from build123d import *

# Parameters (mm, degrees)
SKETCH_1_W          = 30
SKETCH_1_H          = 30
SKETCH_1_W_2        = 28
SKETCH_1_H_2        = 28
EXTRUDE_1_DEPTH     = 225
SKETCH_2_R          = 2
CUT_EXTRUDE_1_DEPTH = 65
SKETCH_4_R          = 2
CUT_EXTRUDE_2_DEPTH = 45
SKETCH_5_R          = 2
CUT_EXTRUDE_3_DEPTH = 45


with BuildPart() as part:
    # 草图1 → 凸台-拉伸1 (new, symmetric)
    with BuildSketch(Plane.XY):
        Rectangle(SKETCH_1_W, SKETCH_1_H)
        Rectangle(SKETCH_1_W_2, SKETCH_1_H_2, mode=Mode.SUBTRACT)
    extrude(amount=EXTRUDE_1_DEPTH, both=True)

    # 草图2 → 切除-拉伸1 (cut, symmetric)
    with BuildSketch(Plane(origin=(15, 0, 0), x_dir=(0, 0, -1), z_dir=(1, 0, 0))):
        with Locations((145.5, 0)):
            Circle(SKETCH_2_R)
        with Locations((170.5, 0)):
            Circle(SKETCH_2_R)
    extrude(amount=CUT_EXTRUDE_1_DEPTH, both=True, mode=Mode.SUBTRACT)

    # 草图4 → 切除-拉伸2 (cut, symmetric)
    with BuildSketch(Plane.XZ.offset(15)):
        with Locations(Location((0, 221, 0), (0, 0, 270))):
            Circle(SKETCH_4_R)
        with Locations(Location((0, 189, 0), (0, 0, 270))):
            Circle(SKETCH_4_R)
    extrude(amount=CUT_EXTRUDE_2_DEPTH, both=True, mode=Mode.SUBTRACT)

    # 草图5 → 切除-拉伸3 (cut, symmetric)
    with BuildSketch(Plane(origin=(15, 0, 0), x_dir=(0, 0, -1), z_dir=(1, 0, 0))):
        with Locations((-221, 0)):
            Circle(SKETCH_5_R)
        with Locations((-189, 0)):
            Circle(SKETCH_5_R)
    extrude(amount=CUT_EXTRUDE_3_DEPTH, both=True, mode=Mode.SUBTRACT)


solid = part.part
The model under review builds one solid part; all positions refer to its coordinate system, in mm. A direction names the side the tool comes from. Coordinates: 2 decimals unless noted, no trailing zeros. Order: outer loops, then holes, each group sorted by start corner. A loop starts at its lowest first (then second) coordinate and runs counter-clockwise, first axis right, second up. Notation, with made-up numbers: (25, -4) -> (55, -4) arc R26 ccw to (55, 20) -> close; hole circle Ø3 at (40, 43). An arc over 180 degrees is marked (long way). Answer in a Markdown table with one row per item.
(1) Machinability: for faces 4 (the flat face through (0, -15, 3)), 5 (the flat face through (0, 14, 3)), which of the approach directions +Z, -Z, +X, -X, +Y, -Y give a long, thin tool a straight path to every point of the face, cutting with its end or side? Answer none if there is none.
Answers:
| item | result |
|---|---|
| face 4 | +Z, -Z, +X, -X, -Y |
| face 5 | +Z, -Z |
(2) The part is to be moulded in two halves that separate along X. For faces 1 (the flat face through (-1.2, -14.4, -225)), 2 (the flat face through (0, -14, 3)), 3 (the flat face through (-15, 0, 3)), say which applies: +X half, -X half, draft (parallel to the pull), parting line (faces both ways), or undercut.
Answers:
| item | result |
|---|---|
| face 1 | draft |
| face 2 | undercut |
| face 3 | -X half |
(3) Consider section A-A (z = 4). Write out the cut boundary in (x, y), plus the area to 3 significant figures.
Answers:
| item | result |
|---|---|
| outline | (-15, -15) -> (15, -15) -> (15, 15) -> (-15, 15) -> close; hole (-14, -14) -> (14, -14) -> (14, 14) -> (-14, 14) -> close |
| area | 116 mm² |
(4) Consider section B-B (x = -9.5). Write out the cut boundary in (y, z), plus the area to 3 significant figures.
Answers:
| item | result |
|---|---|
| outline | (-15, -225) -> (-14, -225) -> (-14, 225) -> (-15, 225) -> close; (14, -225) -> (15, -225) -> (15, 225) -> (14, 225) -> close |
| area | 900 mm² |
(5) Insertion check: pin 1 (10 mm diameter, centred on x = -1.5, y = -7, fed in from -Z). The pin has a flat end and moves straight along its axis. Give the tip position at first contact, or say it passes through.
Answers:
| item | result |
|---|---|
| pin 1 | through |
(6) Wall thickness on line 1 along X through (y, z) = (3.75, -48); line 2 along X through (y, z) = (14.2, 221): over which ranges is each line inside the solid? List them lowest first.
Answers:
| item | result |
|---|---|
| line 1 | -15 to -14, 14 to 15 |
| line 2 | -15 to -2, 2 to 15 |
